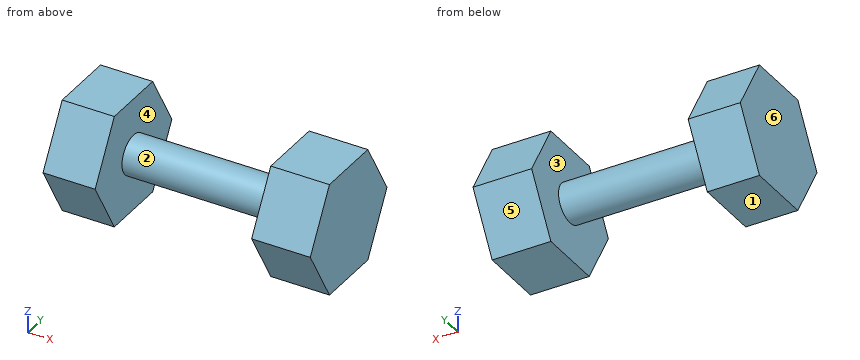
Solid Edge part; units mm, degrees
sketch "Sketch1" plane through (0, 0, 0) normal (1, 0, 0) x (0, 1, 0)
  circle A0 centre (0, 0) radius 15
extrude "Protrusion1" add sketch "Sketch1" along normal mid plane 120
sketch "Sketch2" plane through (-60, 0, 0) normal (-1, 0, 0) x (0, -1, 0)
  line L0 (-25, 43.3013) -> (-50, 0)
  line L1 (-50, 0) -> (-25, -43.3013)
  line L2 (-25, -43.3013) -> (25, -43.3013)
  line L3 (25, -43.3013) -> (50, 0)
  line L4 (50, 0) -> (25, 43.3013)
  line L5 (25, 43.3013) -> (-25, 43.3013)
extrude "ExtrudedProtrusion_2" add sketch "Sketch2" along normal blind 40
sketch "Sketch3" plane through (60, 0, 0) normal (1, 0, 0) x (0, -1, 0)
  line L0 (25, -43.3013) -> (-25, -43.3013)
  line L1 (-25, -43.3013) -> (-50, 0)
  line L2 (-50, 0) -> (-25, 43.3013)
  line L3 (-25, 43.3013) -> (25, 43.3013)
  line L4 (25, 43.3013) -> (50, 0)
  line L5 (50, 0) -> (25, -43.3013)
extrude "Protrusion2" add sketch "Sketch3" along normal blind 45
Design review of the part built by this model. Coordinates are the model's own, in mm. Face numbers are marked on the shaded views. A direction names the side the tool comes from. Coordinates: 2 decimals unless noted, no trailing zeros. Write each loop counter-clockwise with the first axis right and the second up, starting at its lowest first coordinate (ties: lowest second). Pieces come first, ordered by that corner, then holes.
1) Mouldability with a two-part tool opening along X and no side actions: class the marked faces 3, 4, 5 and 6 as +X half, -X half, draft (parallel to the pull), parting line (faces both ways), or undercut.
2) Add section B-B (z = 31). Write out the cut boundary in (x, y).
3) Insertion check: pin 1 (3 mm diameter, centred on x = 3, z = 1, fed in from +Y); pin 2 (2 mm diameter, centred on x = 72.5, z = 16, fed in from -Y); pin 3 (5 mm diameter, centred on x = -73, y = 37.5, fed in from -Z). Each pin has a flat end and moves straight along its axis. Give the tip position at first contact, or say it passes through.
4) Add section D-D (x = -79.5). Write out the cut boundary in (y, z), plus the area to 3 significant figures.
5) Machinability: for the marked faces 1 and 2, which of the approach directions +Z, -Z, +X, -X, +Y, -Y give a long, thin tool a straight path to every point of the face, cutting with its end or side? Answer none if there is none.
6) Add section C-C (y = 0). Write out the cut boundary in (x, z).
7) Add section A-A (y = 18). Write out the cut boundary in (x, z).
8) To check wall thickness, follow L1, parallel to X at y = 12, z = 38; L2, parallel to Z at x = 23, y = 9.5; L3, parallel to Y at x = -79, z = -3. State the ranges of each line that lie inside material, in increasing order.
Check result:
1. face 3: undercut
1. face 4: undercut
1. face 5: draft
1. face 6: -X half
2. outline: (-100, -32.1) - (-60, -32.1) - (-60, 32.1) - (-100, 32.1) - close; (60, -32.1) - (105, -32.1) - (105, 32.1) - (60, 32.1) - close
3. pin 1: stops at y = 15
3. pin 2: stops at y = -41.34
3. pin 3: stops at z = -25.98
4. outline: (-50, 0) - (-25, -43.3) - (25, -43.3) - (50, 0) - (25, 43.3) - (-25, 43.3) - close
4. area: 6,500 mm2
5. face 1: -Z, +X, -X, +Y, -Y
5. face 2: none
6. outline: (-100, -43.3) - (-60, -43.3) - (-60, -15) - (60, -15) - (60, -43.3) - (105, -43.3) - (105, 43.3) - (60, 43.3) - (60, 15) - (-60, 15) - (-60, 43.3) - (-100, 43.3) - close
7. outline: (-100, -43.3) - (-60, -43.3) - (-60, 43.3) - (-100, 43.3) - close; (60, -43.3) - (105, -43.3) - (105, 43.3) - (60, 43.3) - close
8. L1: x = -100 to -60, 60 to 105
8. L2: z = -11.61 to 11.61
8. L3: y = -48.27 to 48.27
